```python
from build123d import *

# Parameters (mm, degrees)
ESQUISSE2_R        = 1.35
BOSS_EXTRU_2_DEPTH = 6


with BuildPart() as part:
    # Esquisse1 → Révolution1 (revolve)
    with BuildSketch(Plane.XY, mode=Mode.PRIVATE) as r_volution1_sk:
        Polygon((-6.05, 0), (-6.05, 4), (-3.85, 4), (-3.25, 4.6), (-3.25, 25.8), (-3.85, 26.4), (-6.05, 26.4), (-6.05, 30.4), (-8, 30.4), (-8, 24.4), (-5, 21.4), (-5, 9), (-8, 6), (-8, 0), align=None)
    revolve(r_volution1_sk.sketch.rotate(Axis((0, -1.144220684, 0), (0, 1, 0)), 270), axis=Axis((0, -1.144220684, 0), (0, 1, 0)))

    # Esquisse2 → Boss.-Extru.2 (add)
    with BuildSketch(Plane(origin=(0, 0, 0), x_dir=(1, 0, 0), z_dir=(0, 1, 0))):
        with BuildLine():
            Line((-7.878088106, -1.391304348), (-3.939044053, -23.695652174))
            ThreePointArc((-3.939044053, -23.695652174), (0, -27), (3.939044053, -23.695652174))
            Line((3.939044053, -23.695652174), (7.878088106, -1.391304348))
            ThreePointArc((7.878088106, -1.391304348), (0, -8), (-7.878088106, -1.391304348))
        make_face()
        with Locations(Location((0, -23, 0), (0, 0, 270))):
            Circle(ESQUISSE2_R, mode=Mode.SUBTRACT)
    extrude(amount=BOSS_EXTRU_2_DEPTH)


solid = part.part
```
Part model, mm, in its own coordinate system. A direction names the side the tool comes from. Round coordinates to 2 decimals unless told otherwise and drop trailing zeros. Order: outer loops, then holes, each group sorted by start corner. A loop starts at its lowest first (then second) coordinate and runs counter-clockwise, first axis right, second up. Notation, with made-up numbers: M -12,41.25 L 13,41.25 A24 cw 13,59.25 Z; hole C 21,83.5 d8. An arc over 180 degrees is marked long. Answer in a Markdown table with one row per item. Add a question column.
Q1. Cut at B-B on z = 0. Give the cut face in (x, y), and give its area (3 significant figures).
Q2. Cut at D-D on y = 22. Give the cut face in (x, z).
Q3. 3-axis set-ups, long thin cutter, end or side, ignore diameter. For faces 1 (the face through (-1.82, 28.43, -5.77)), 2 (the face through (0, 3, 27)), 3 (the face through (5.064, 8.812, 1.125)), 4 (the face through (-1.82, 2.03, -5.77)): which of +Z, -Z, +X, -X, +Y, -Y reach the whole face in a straight line?
Q4. Mould opens along Y. For faces 5 (the face through (4.88, 15.11, 1.08)), 6 (the face through (-6, 30.4, -2)), 7 (the face through (5.88, 2.96, 12.7)), 8 (the face through (0, 0, 10)) say: +Y half, -Y half, draft (parallel to the pull), parting line (faces both ways), or undercut.
Q5. Cut at A-A on x = 0. Give the number of separate pieces and of enclosed holes in the cut face, and give its area (3 significant figures).
Q6. Cut at C-C on y = 3. Give the cut face in (x, z).
Q7. Pin check, flat tips, straight feed: pin 1 (3.5 mm diameter, centred on x = 1.5, z = -0.5, fed in from +Y); pin 2 (8 mm diameter, centred on x = 3.5, z = 19, fed in from +Y); pin 3 (2.5 mm diameter, centred on x = 0, z = 23, fed in from -Y); pin 4 (8 mm diameter, centred on y = 8.5, z = 7.5, fed in from +X). Stop position of each tip, or through.
Q8. Wall check: L1, parallel to X at y = 1, z = 0; L2, parallel to X at y = 20, z = 0; L3, parallel to Y at x = 5, z = 7. Give the ranges that are in metal, low to high. Write a range as from..to.
Established:
| question | item | result |
|---|---|---|
| 1 | outline | M -8,0 L -6.05,0 L -6.05,4 L -3.85,4 L -3.25,4.6 L -3.25,25.8 L -3.85,26.4 L -6.05,26.4 L -6.05,30.4 L -8,30.4 L -8,24.4 L -5,21.4 L -5,9 L -8,6 Z; M 3.25,4.6 L 3.85,4 L 6.05,4 L 6.05,0 L 8,0 L 8,6 L 5,9 L 5,21.4 L 8,24.4 L 8,30.4 L 6.05,30.4 L 6.05,26.4 L 3.85,26.4 L 3.25,25.8 Z |
| 1 | area | 151 mm2 |
| 2 | outline | C 0,0 d11.2; hole C 0,0 d6.5 |
| 3 | face 1 | +Y |
| 3 | face 2 | +Z, +Y, -Y |
| 3 | face 3 | none |
| 3 | face 4 | -Y |
| 4 | face 5 | undercut |
| 4 | face 6 | +Y half |
| 4 | face 7 | draft |
| 4 | face 8 | -Y half |
| 5 | separate pieces | 3 |
| 5 | enclosed holes | 0 |
| 5 | area | 249 mm2 |
| 6 | outline | M -7.88,1.39 A8 ccw long 7.88,1.39 L 3.94,23.7 A4 ccw -3.94,23.7 Z; hole C 0,0 d12.1; hole C 0,23 d2.7 |
| 7 | pin 1 | stops at y = 25.88 |
| 7 | pin 2 | stops at y = 6 |
| 7 | pin 3 | passes through |
| 7 | pin 4 | stops at x = 7.35 |
| 8 | L1 | x = -8..-6.05, 6.05..8 |
| 8 | L2 | x = -5..-3.25, 3.25..5 |
| 8 | L3 | y = 0..6 |
